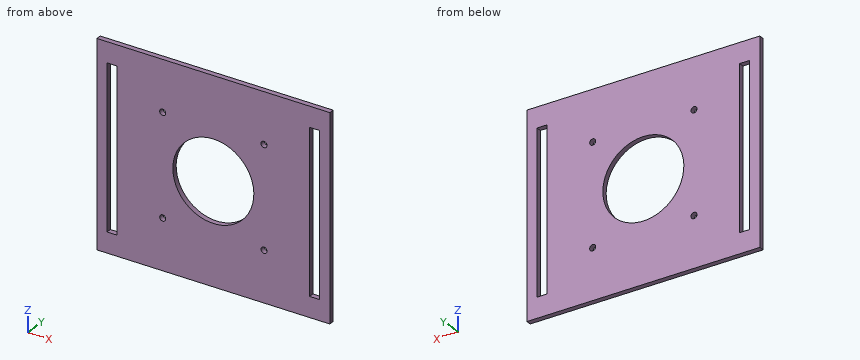
from build123d import *

# Parameters (mm, degrees)
SKETCH1_W           = 230
SKETCH1_H           = 200
SKETCH1_W_2         = 10
SKETCH1_H_2         = 160
BOSS_EXTRUDE1_DEPTH = 5
SKETCH2_R           = 40
SKETCH2_R_2         = 3
CUT_EXTRUDE1_DEPTH  = 5


with BuildPart() as part:
    # Sketch1 → Boss-Extrude1 (new body)
    with BuildSketch(Plane(origin=(0, 0, 0), x_dir=(1, 0, 0), z_dir=(0, 1, 0))):
        Rectangle(SKETCH1_W, SKETCH1_H)
        with Locations((-100, 0)):
            Rectangle(SKETCH1_W_2, SKETCH1_H_2, mode=Mode.SUBTRACT)
        with Locations((100, 0)):
            Rectangle(SKETCH1_W_2, SKETCH1_H_2, mode=Mode.SUBTRACT)
    extrude(amount=BOSS_EXTRUDE1_DEPTH)

    # Sketch2 → Cut-Extrude1 (cut)
    with BuildSketch(Plane(origin=(0, 5, 0), x_dir=(1, 0, 0), z_dir=(0, 1, 0))):
        with Locations(Location((0, 0, 0), (0, 0, 270))):
            Circle(SKETCH2_R)
        with Locations(Location((-50, 50, 0), (0, 0, 270))):
            Circle(SKETCH2_R_2)
        with Locations(Location((50, 50, 0), (0, 0, 270))):
            Circle(SKETCH2_R_2)
        with Locations(Location((50, -50, 0), (0, 0, 270))):
            Circle(SKETCH2_R_2)
        with Locations(Location((-50, -50, 0), (0, 0, 270))):
            Circle(SKETCH2_R_2)
    extrude(amount=-CUT_EXTRUDE1_DEPTH, mode=Mode.SUBTRACT)


solid = part.part
Check sheet for the modelled part. Datum: model origin and axes. Units: mm. Round coordinates to 2 decimals unless told otherwise and drop trailing zeros. Order: outer loops, then holes, each group sorted by start corner. A loop starts at its lowest first (then second) coordinate and runs counter-clockwise, first axis right, second up.
(1) Scan lines: probe 1 along X at (y, z) = (1.8, 42.5); probe 2 along X at (y, z) = (2.45, 50); probe 3 along Z at (x, y) = (-96, 3.9). Record each from-to range of solid material in increasing order.
(2) Cross-section at C-C, the plane x = 50. Enter the section's corners in (y, z), and give its area (3 significant figures).
(3) Cross-section at A-A, the plane x = 0. Enter the section's corners in (y, z), and give its area (3 significant figures).
(4) Go/stop test with a flat-tipped pin: P1, Ø3.5, axis at x = -50, z = 50, coming from the +Y side. Record where the tip stops, or that it passes through.
(5) Cross-section at D-D, the plane y = 2.5. Enter the section's corners in (x, z).
(6) Cross-section at B-B, the plane z = 50. Enter the section's corners in (x, y).
Check sheet entries:
1. probe 1: x = -115 to -105, -95 to 95, 105 to 115
1. probe 2: x = -115 to -105, -95 to -53, -47 to 47, 53 to 95, 105 to 115
1. probe 3: z = -100 to -80, 80 to 100
2. outline: (0, -100) - (5, -100) - (5, -53) - (0, -53) - close; (0, -47) - (5, -47) - (5, 47) - (0, 47) - close; (0, 53) - (5, 53) - (5, 100) - (0, 100) - close
2. area: 940 mm2
3. outline: (0, -100) - (5, -100) - (5, -40) - (0, -40) - close; (0, 40) - (5, 40) - (5, 100) - (0, 100) - close
3. area: 600 mm2
4. P1: passes through
5. outline: (-115, -100) - (115, -100) - (115, 100) - (-115, 100) - close; hole (-105, -80) - (-95, -80) - (-95, 80) - (-105, 80) - close; hole circle Ø6 at (-50, -50); hole circle Ø6 at (-50, 50); hole circle Ø80 at (0, 0); hole circle Ø6 at (50, -50); hole circle Ø6 at (50, 50); hole (95, -80) - (105, -80) - (105, 80) - (95, 80) - close
6. outline: (-115, 0) - (-105, 0) - (-105, 5) - (-115, 5) - close; (-95, 0) - (-53, 0) - (-53, 5) - (-95, 5) - close; (-47, 0) - (47, 0) - (47, 5) - (-47, 5) - close; (53, 0) - (95, 0) - (95, 5) - (53, 5) - close; (105, 0) - (115, 0) - (115, 5) - (105, 5) - close
